Input: part model. Units: mm. Frame: model coordinates. Face numbers are marked on the shaded views. A direction names the side the tool comes from. Coordinates: 2 decimals unless noted, no trailing zeros. Order: outer loops, then holes, each group sorted by start corner. A loop starts at its lowest first (then second) coordinate and runs counter-clockwise, first axis right, second up. Notation, with made-up numbers: (-14, 55.5) - (45, 55.5) arc R12 cw to (45, 69.5) - close; hole circle Ø9 at (2, 14). An arc over 180 degrees is marked (long way). Use a Markdown table: item, result. Add a question column.
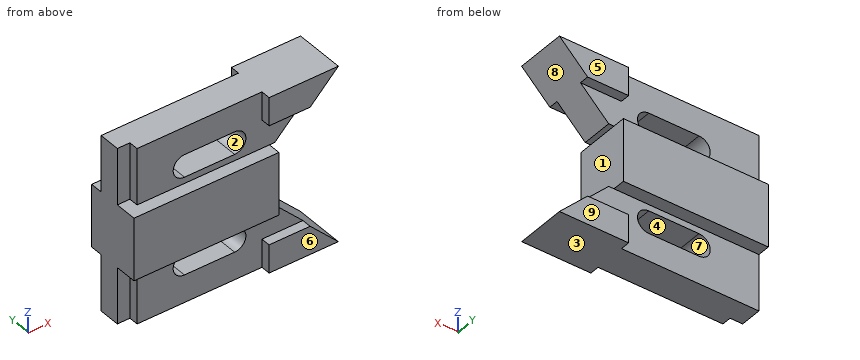
from build123d import *

# Parameters (mm, degrees)
F1_DEPTH = 14.224
F2_DEPTH = 12.7
F3_DEPTH = 7.874
F0_W     = 6.35
F0_H     = 28.575
F4_DEPTH = 7.874
F5_DEPTH = 3.048


with BuildPart() as f1:
    # F0 (on Front) → F1 (new body, symmetric)
    with BuildSketch(Plane.XZ):
        Polygon((-45.974, 0), (-52.324, 0), (-52.324, -15.875), (21.082, -15.875), (21.082, 0), align=None)
    extrude(amount=F1_DEPTH, both=True)



with BuildPart() as f2:
    # F0 (on Front) → F2 (new body, symmetric)
    with BuildSketch(Plane.XZ):
        Polygon((52.324, 28.575), (17.272, 28.575), (17.272, 14.2875), (38.0365, 14.2875), align=None)
    extrude(amount=F2_DEPTH, both=True)


with BuildPart() as f1_1:
    add(f1.part)

    add(f2.part)  # F3 merges F2
    # F0 (on Front) → F3 (join, symmetric)
    with BuildSketch(Plane.XZ):
        Polygon((17.272, 28.575), (-45.974, 28.575), (-45.974, 0), (21.082, 0), (23.749, 0), (38.0365, 14.2875), (17.272, 14.2875), align=None)
        with BuildLine():
            ThreePointArc((-21.971, 3.175), (-27.686, 8.89), (-21.971, 14.605))
            Line((-21.971, 14.605), (3.429, 14.605))
            ThreePointArc((3.429, 14.605), (9.144, 8.89), (3.429, 3.175))
            Line((3.429, 3.175), (-21.971, 3.175))
        make_face(mode=Mode.SUBTRACT)
    extrude(amount=F3_DEPTH, both=True)

    # F0 (on Front) → F4 (join)
    with BuildSketch(Plane.XZ):
        with Locations((-49.149, 14.2875)):
            Rectangle(F0_W, F0_H)
    extrude(amount=-F4_DEPTH)

    # F0 (on Front) → F5 (join)
    with BuildSketch(Plane.XZ):
        with Locations((-49.149, 14.2875)):
            Rectangle(F0_W, F0_H)
    extrude(amount=F5_DEPTH)

    # F6: F1 across face


with BuildPart() as f1_2:
    add(f1_1.part)
    add(f1_1.part.mirror(Plane(origin=(-15.621, 0, -15.875), x_dir=(1, 0, 0), z_dir=(0, 0, -1))))


solid = f1_2.part
1) Cut plane B-B (z = -40.64). Return the cut outline in (x, y), and give its area (3 significant figures).
2) Reachability of the marked faces 5, 6, 7, 8 and 9 from +Z, -Z, +X, -X, +Y, -Y: full face, straight path, thin tool, end or side. Return the list, or none.
3) Cut plane C-C (x = 0). Return the cut outline in (y, z) (3 decimals).
4) Cut plane A-A (y = 10). State how many separate pieces and enclosed holes the cut face has, and give its area (3 significant figures).
5) Material intervals for L1, parallel to Z at x = 3.5, y = -6 (3 decimals); L2, parallel to X at y = -1.25, z = -11; L3, parallel to Z at x = 22.5, y = -5.75 (3 decimals), sorted ascending.
6) Contact query for flat-ended pins moving along their axis: P1, Ø2, axis at y = -4, z = -43, coming from the +X side; P2, Ø1.4, axis at y = 9.5, z = -51, coming from the -X side; P3, Ø11.5, axis at x = 30.5, z = -50, coming from the +Y side. Output: stop coordinate, or through.
7) Pull-direction query (X, two-part tool) for the marked faces 1, 2, 3 and 4; classes: pulls with the +X half, pulls with the -X half, needs draft (parallel to the pull), parting line crosses it, or undercut.
Computed:
| question | item | result |
|---|---|---|
| 1 | outline | (-52.32, -3.05) - (-45.97, -3.05) - (-45.97, -7.87) - (-27.69, -7.87) - (-27.69, 7.87) - (-52.32, 7.87) - close; (9.14, -7.87) - (32.64, -7.87) - (32.64, 7.87) - (9.14, 7.87) - close |
| 1 | area | 727 mm2 |
| 2 | face 5 | +Z, +X, -X, +Y |
| 2 | face 6 | -Z, +X, -X, -Y |
| 2 | face 7 | +Y, -Y |
| 2 | face 8 | +X, +Y, -Y |
| 2 | face 9 | -Z, +X, -X, +Y |
| 3 | outline | (-14.224, -31.75) - (-7.874, -31.75) - (-7.874, -34.925) - (7.874, -34.925) - (7.874, -31.75) - (14.224, -31.75) - (14.224, 0) - (7.874, 0) - (7.874, 3.175) - (-7.874, 3.175) - (-7.874, 0) - (-14.224, 0) - close; (-7.874, -60.325) - (7.874, -60.325) - (7.874, -46.355) - (-7.874, -46.355) - close; (-7.874, 14.605) - (7.874, 14.605) - (7.874, 28.575) - (-7.874, 28.575) - close |
| 4 | separate pieces | 3 |
| 4 | enclosed holes | 0 |
| 4 | area | 3,130 mm2 |
| 5 | L1 | z = -60.325 to -46.355, -34.925 to 3.175, 14.605 to 28.575 |
| 5 | L2 | x = -52.32 to 21.08 |
| 5 | L3 | z = -60.325 to -31.75, 0 to 28.575 |
| 6 | P1 | stops at x = 36 |
| 6 | P2 | stops at x = 17.27 |
| 6 | P3 | stops at y = 12.7 |
| 7 | face 1 | pulls with the +X half |
| 7 | face 2 | undercut |
| 7 | face 3 | needs draft |
| 7 | face 4 | undercut |
